from build123d import *

# Parameters (mm, degrees)
SKETCH1_R           = 52.5
BOSS_EXTRUDE1_DEPTH = 20
SKETCH2_R           = 42.5
SKETCH2_R_2         = 40
CUT_EXTRUDE1_DEPTH  = 10
SKETCH4_R           = 40
CUT_EXTRUDE3_DEPTH  = 10
SKETCH8_R           = 55
CUT_EXTRUDE4_DEPTH  = 7.5
SKETCH9_R           = 37.5
CUT_EXTRUDE5_DEPTH  = 2.5
FILLET1_R           = 5
SKETCH10_R          = 2.5
CUT_EXTRUDE6_DEPTH  = 5
SKETCH11_R          = 1.5
CUT_EXTRUDE7_DEPTH  = 7.5
SKETCH13_R          = 1.5
CUT_EXTRUDE9_DEPTH  = 7.5
SKETCH14_R          = 1.5
CUT_EXTRUDE10_DEPTH = 7.5
SKETCH15_R          = 1.5
CUT_EXTRUDE11_DEPTH = 7.5


with BuildPart() as part:
    # Sketch1 → Boss-Extrude1 (new body)
    with BuildSketch(Plane.XY):
        Circle(SKETCH1_R)
    extrude(amount=BOSS_EXTRUDE1_DEPTH)

    # Sketch2 → Cut-Extrude1 (cut)
    with BuildSketch(Plane(origin=(0, 0, 0), x_dir=(-1, 0, 0), z_dir=(0, 0, -1))):
        Circle(SKETCH2_R)
        Circle(SKETCH2_R_2, mode=Mode.SUBTRACT)
    extrude(amount=-CUT_EXTRUDE1_DEPTH, mode=Mode.SUBTRACT)

    # Sketch4 → Cut-Extrude3 (cut)
    with BuildSketch(Plane(origin=(0, 0, 0), x_dir=(-1, 0, 0), z_dir=(0, 0, -1))):
        Circle(SKETCH4_R)
    extrude(amount=-CUT_EXTRUDE3_DEPTH, mode=Mode.SUBTRACT)

    # Sketch8 → Cut-Extrude4 (cut)
    with BuildSketch(Plane.XY.offset(20)):
        Circle(SKETCH8_R)
    extrude(amount=-CUT_EXTRUDE4_DEPTH, mode=Mode.SUBTRACT)

    # Sketch9 → Cut-Extrude5 (cut)
    with BuildSketch(Plane(origin=(0, 0, 10), x_dir=(-1, 0, 0), z_dir=(0, 0, -1))):
        Circle(SKETCH9_R)
    extrude(amount=-CUT_EXTRUDE5_DEPTH, mode=Mode.SUBTRACT)

    # Fillet1
    fillet1_edges = [part.edges().sort_by_distance(p)[0] for p in [
        (-52.5, 0, 12.5),
    ]]
    fillet(fillet1_edges, radius=FILLET1_R)

    # Sketch10 → Cut-Extrude6 (cut)
    with BuildSketch(Plane.XY.offset(12.5)):
        with Locations((0, 46.25)):
            Circle(SKETCH10_R)
        with Locations((46.25, 0)):
            Circle(SKETCH10_R)
        with Locations((0, -46.25)):
            Circle(SKETCH10_R)
        with Locations((-46.25, 0)):
            Circle(SKETCH10_R)
    extrude(amount=-CUT_EXTRUDE6_DEPTH, mode=Mode.SUBTRACT)

    # Sketch11 → Cut-Extrude7 (cut)
    with BuildSketch(Plane.XY.offset(7.5)):
        with Locations((0, 46.25)):
            Circle(SKETCH11_R)
    extrude(amount=-CUT_EXTRUDE7_DEPTH, mode=Mode.SUBTRACT)

    # Sketch13 → Cut-Extrude9 (cut)
    with BuildSketch(Plane.XY.offset(7.5)):
        with Locations((0, -46.25)):
            Circle(SKETCH13_R)
    extrude(amount=-CUT_EXTRUDE9_DEPTH, mode=Mode.SUBTRACT)

    # Sketch14 → Cut-Extrude10 (cut)
    with BuildSketch(Plane.XY.offset(7.5)):
        with Locations((-46.25, 0)):
            Circle(SKETCH14_R)
    extrude(amount=-CUT_EXTRUDE10_DEPTH, mode=Mode.SUBTRACT)

    # Sketch15 → Cut-Extrude11 (cut)
    with BuildSketch(Plane.XY.offset(7.5)):
        with Locations((46.25, 0)):
            Circle(SKETCH15_R)
    extrude(amount=-CUT_EXTRUDE11_DEPTH, mode=Mode.SUBTRACT)


solid = part.part
Can you work these out from the model? Positions are in its coordinate system, mm. A direction names the side the tool comes from. Coordinates: 2 decimals unless noted, no trailing zeros. Write each loop counter-clockwise with the first axis right and the second up, starting at its lowest first coordinate (ties: lowest second). Pieces come first, ordered by that corner, then holes. Notation, with made-up numbers: (50.5, 71) -> (75.5, 71) arc R21 ccw to (75.5, 95) -> close; hole circle Ø1 at (69, 59.25). An arc over 180 degrees is marked (long way). Write each question's results on one line, items separated by ' | '. Start each with the question number.
Q1. I'm going to push flat-ended pins straight in: pin 1 (1.5 mm diameter, centred on y = 10.5, z = 5, fed in from +X); pin 2 (4 mm diameter, centred on y = 39, z = 10.5, fed in from +X); pin 3 (1.5 mm diameter, centred on x = -46, y = -0.5, fed in from +Z); pin 4 (2 mm diameter, centred on x = 33, z = 10.5, fed in from -Y). Where does each tip first touch, or does it pass through?
Q2. If I drill on probe 1 along Y at (x, z) = (0, 3.25); probe 2 along Y at (x, z) = (-1.5, 11); probe 3 along Z at (x, y) = (-8, -41), over which ranges is the centre line in solid material (lowest first)?
Q3. Imagine slicing it at B-B (z = 5.5). Write out the boundary of the cut face in (x, y), then the cut area to 3 significant figures.
Q4. We'd pull the mould along X, two halves only. Please class faces 4 (the face through (43, -4, 0)), 5 (the face through (-0.5, -48.7, 10)), 6 (the face through (50.076, 15.77, 3.698)): +X half, -X half, draft (parallel to the pull), parting line (faces both ways), or undercut.
Q5. Imagine slicing it at A-A (x = 0). Write out the boundary of the cut face in (y, z), then the cut area to 3 significant figures.
Q6. On a 3-axis mill with a long thin cutter (end or side, diameter ignored), from which of +Z, -Z, +X, -X, +Y, -Y can I reach the whole of each face in a straight line? I mean faces 1 (the face through (-0.5, 43.8, 10)), 2 (the face through (33.727, -25.861, 4.93)), 3 (the face through (-0.325, -47.714, 3.802)). Say none if no direction works.
Taken from the geometry:
1) pin 1: stops at x = 51.59 | pin 2: stops at x = 36.38 | pin 3: passes through | pin 4: stops at y = -40.69
2) probe 1: y = -52.5 to -47.75, -44.75 to -42.5, 42.5 to 44.75, 47.75 to 52.5 | probe 2: y = -51.05 to -48.25, -44.25 to -37.47, 37.47 to 44.25, 48.25 to 51.05 | probe 3: z = 10 to 12.5
3) outline: circle Ø105 at (0, 0); hole circle Ø3 at (-46.25, 0); hole circle Ø85 at (0, 0); hole circle Ø3 at (0, -46.25); hole circle Ø3 at (0, 46.25); hole circle Ø3 at (46.25, 0) | area: 2,960 mm^2
4) face 4: draft | face 5: undercut | face 6: parting line
5) outline: (-52.5, 0) -> (-47.75, 0) -> (-47.75, 7.5) -> (-48.75, 7.5) -> (-48.75, 12.34) arc R5 ccw to (-52.5, 7.5) -> close; (-44.75, 0) -> (-42.5, 0) -> (-42.5, 10) -> (-37.5, 10) -> (-37.5, 12.5) -> (-43.75, 12.5) -> (-43.75, 7.5) -> (-44.75, 7.5) -> close; (37.5, 10) -> (42.5, 10) -> (42.5, 0) -> (44.75, 0) -> (44.75, 7.5) -> (43.75, 7.5) -> (43.75, 12.5) -> (37.5, 12.5) -> close; (47.75, 0) -> (52.5, 0) -> (52.5, 7.5) arc R5 ccw to (48.75, 12.34) -> (48.75, 7.5) -> (47.75, 7.5) -> close | area: 169 mm^2
6) face 1: +Z | face 2: -Z | face 3: +Z, -Z
